from build123d import *

# Parameters (mm, degrees)
GAGE_PLATE_SIDE_EXTRUDE_DEPTH = 3.175
BOSS_EXTRUDE2_DEPTH           = 76.2
FILLET1_R                     = 2.54
FILLET2_R                     = 7.62


with BuildPart() as part:
    # Sketch1 → Gage Plate-side Extrude (new body)
    with BuildSketch(Plane(origin=(0, 0, 0), x_dir=(1, 0, 0), z_dir=(0, 1, 0))):
        Polygon((0, 0), (0, -12.7), (-30.463396962, -12.7), (-56.042370913, -8.189736754), (-84.03796246, 1.99982526), (-86.502886868, 12.65434565), (-56.042370913, 1.567624522), align=None)
    extrude(amount=GAGE_PLATE_SIDE_EXTRUDE_DEPTH)

    # Sketch2 → Boss-Extrude2 (add)
    with BuildSketch(Plane(origin=(0, 3.175, 0), x_dir=(1, 0, 0), z_dir=(0, 1, 0))):
        Polygon((0, 0), (0, -2.344295335), (-56.042370913, -0.776670813), (-85.910666223, 10.094499628), (-86.502886868, 12.65434565), (-56.042370913, 1.567624522), align=None)
    extrude(amount=BOSS_EXTRUDE2_DEPTH)

    # Fillet1
    # the kernel refuses this fillet: 2.54 mm, written as the material it takes off along each edge
    with BuildSketch(Plane(origin=(-30.463396962, -0.555553013, 12.7), x_dir=(-0.9848077530122088, 0, -0.17364817766692622), z_dir=(0, 1, 0)), Plane(origin=(-56.042370913, -0.555553013, 8.189736754), x_dir=(-0.9396926207859081, 0, -0.3420201433256695), z_dir=(0, 1, 0))) as fillet1_piece_1:
        with BuildLine():
            CenterArc((FILLET1_R * 0.0874886635259, -FILLET1_R), FILLET1_R, 90, 10)
            Line((-FILLET1_R * 0.086159514141, -FILLET1_R * 0.0151922469878), (0, 0))
            Line((0, 0), (FILLET1_R * 0.0874886635259, 0))
        make_face()
    extrude(amount=4.286106027, mode=Mode.SUBTRACT)
    with BuildSketch(Plane(origin=(-56.042370913, 3.175, 0.776670813), x_dir=(-0.9396926207859059, 0, -0.3420201433256751), z_dir=(0, 1, 0))) as fillet1_piece_2:
        with BuildLine():
            CenterArc((FILLET1_R * 0.161944353893, -FILLET1_R), FILLET1_R, 90, 18.397732774)
            Line((-FILLET1_R * 0.153667135261, -FILLET1_R * 0.0511114986921), (0, 0))
            Line((0, 0), (FILLET1_R * 0.161944353893, 0))
        make_face()
    extrude(amount=77.228346647, mode=Mode.SUBTRACT)
    with BuildSketch(Plane(origin=(0, 3.175, 2.344295335), x_dir=(0, 0, -1), z_dir=(0, 1, 0))) as fillet1_piece_3:
        with BuildLine():
            CenterArc((2.611648042, 2.525890443), FILLET1_R, 178.397732774, 85.560295248)
            Line((0.072641158, 2.596911875), (0, 0))
            Line((0, 0), (2.344295335, 0))
        make_face()
    extrude(amount=82.694819102, mode=Mode.SUBTRACT)
    with BuildSketch(Plane(origin=(-85.910666223, 3.175, -10.094499628), x_dir=(-0.22539678463569066, 0, -0.9742670524429594), z_dir=(0, 1, 0))) as fillet1_piece_4:
        with BuildLine():
            CenterArc((FILLET1_R * 0.542659564301, -FILLET1_R), FILLET1_R, 90, 56.973788384)
            Line((-FILLET1_R * 0.295761754969, -FILLET1_R * 0.454977347815), (0, 0))
            Line((0, 0), (FILLET1_R * 0.542659564301, 0))
        make_face()
    extrude(amount=79.645888233, mode=Mode.SUBTRACT)

    # Fillet2
    fillet2_edges = [part.edges().sort_by_distance(p)[0] for p in [
        (0, 1.5875, 12.7),
        (-84.03796246, 1.5875, -1.99982526),
    ]]
    fillet(fillet2_edges, radius=FILLET2_R)


solid = part.part
Work out the finished part from the listing and answer in its coordinate system (mm). A direction names the side the tool comes from. Give positions to 0.01 mm unless a question says otherwise; leave off trailing zeros. Loops run counter-clockwise (first coordinate to the right, second up) from the corner with the lowest first, then second, coordinate; pieces in that order, holes last. Notation, with made-up numbers: (83, 72) -> (90, 72) arc R30 ccw to (90, 96) -> close; hole circle Ø6 at (6.5, 31). An arc over 180 degrees is marked (long way). Use a Markdown table: item, result. Add a question column.
1) The part is cut by section D-D, the plane x = -14. Determine the outline of the cut face in (y, z) (3 decimals), plus the area to 3 significant figures.
2) Which of the six approach directions +Z, -Z, +X, -X, +Y, -Y give full straight-line access (tool end or side, diameter ignored) to faces 1 (the cylindrical face through (-2.291, 1.61, 10.527)), 2 (the flat face through (-70.32, 40.74, -4.42))?
3) Consider line 1 along Y through (x, z) = (-27.5, 6) (3 decimals); line 2 along Z through (x, y) = (-33.5, 22.5); line 3 along Z through (x, y) = (-25, 72.5) (3 decimals). Determine where each line is inside the solid, lowest interval first.
4) The part is cut by section C-C, the plane z = 3.5. Determine the outline of the cut face in (x, y) (3 decimals), plus the area to 3 significant figures.
5) The part is cut by section B-B, the plane x = -24.5. Determine the outline of the cut face in (y, z) (3 decimals), plus the area to 3 significant figures.
6) The part is cut by section A-A, the plane y = 56. Determine the outline of the cut face in (x, z).
7) Each of these flat-tipped pins is pushed along its axis until it touches: P1, Ø3, axis at x = -72, y = 51, coming from the -Z side; P2, Ø8, axis at x = -12.5, z = -2.5, coming from the -Y side; P3, Ø10, axis at y = 46, z = -7.5, coming from the -X side; P4, Ø10, axis at y = 16.5, z = 7, coming from the +X side. Where does it stop, or does it pass through?
Reported:
| question | item | result |
|---|---|---|
| 1 | outline | (0, -0.392) -> (79.375, -0.392) -> (79.375, 1.953) -> (3.175, 1.953) -> (3.175, 12.7) -> (0, 12.7) -> close |
| 1 | area | 220 mm^2 |
| 2 | face 1 | +Z, +X, +Y, -Y |
| 2 | face 2 | +Z, -X, +Y |
| 3 | line 1 | y = 0 to 3.175 |
| 3 | line 2 | z = -0.94 to 1.41 |
| 3 | line 3 | z = -0.699 to 1.645 |
| 4 | outline | (-68.927, 0) -> (0, 0) -> (0, 3.175) -> (-68.927, 3.175) -> close |
| 4 | area | 219 mm^2 |
| 5 | outline | (0, -0.685) -> (79.375, -0.685) -> (79.375, 1.659) -> (3.175, 1.659) -> (3.175, 12.7) -> (0, 12.7) -> close |
| 5 | area | 221 mm^2 |
| 6 | outline | (-86.5, -12.65) -> (-56.04, -1.57) -> (0, 0) arc R2.54 ccw to (-2.6, 2.27) -> (-55.63, 0.79) arc R2.54 ccw to (-56.43, 0.64) -> (-84.62, -9.62) arc R2.54 ccw to (-86.22, -11.44) -> close |
| 7 | P1 | stops at z = -7.92 |
| 7 | P2 | stops at y = 0 |
| 7 | P3 | stops at x = -86.47 |
| 7 | P4 | stops at x = -1.38 |
